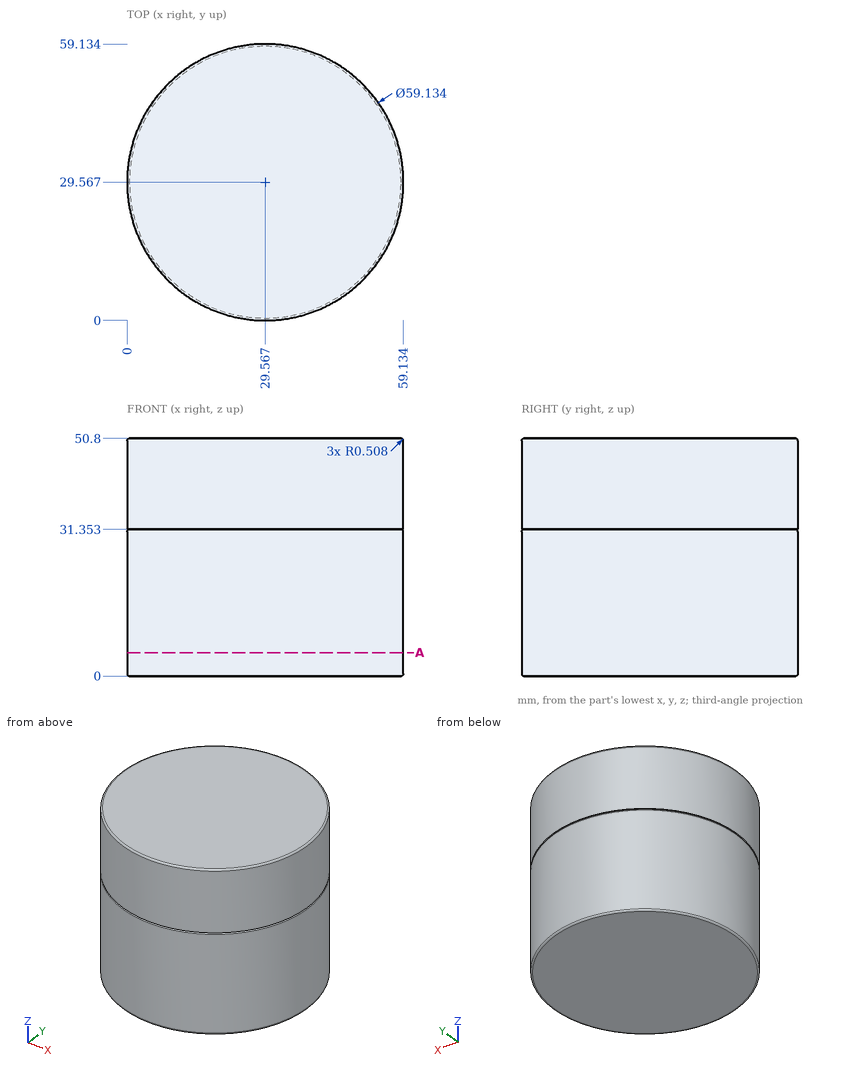
The drawing under review shows one solid part. Ordinate dimensions are in mm from its lowest x, y, z. Give positions to 0.01 mm unless a question says otherwise; leave off trailing zeros. Loops run counter-clockwise (first coordinate to the right, second up) from the corner with the lowest first, then second, coordinate; pieces in that order, holes last. Notation, with made-up numbers: M 87.5,-16 L 92.5,-16 A11 cw 92.5,-11 Z; hole C 44,-23.5 d7. An arc over 180 degrees is marked long. One line per item, written item: value. Start each with the question number.
Q1. For L1, parallel to X at y = 23.5, z = 39.5 (1 decimal); L2, parallel to Y at x = 41, z = 6 (1 decimal); L3, parallel to Y at x = 27, z = 19, list the stretches that pass through material, from the lowest coordinate up.
Q2. Add section A-A (z = 5). Give the boundary of the cut face in (x, y) (1 decimal).
Q3. Clearance check with flat-ended pins moving along their axes: pin 1 Ø12 at (y, z) = (44, 7.5) entering from -X; pin 2 Ø4 at (y, z) = (39.5, 25) entering from +X; pin 3 Ø12 at (x, z) = (48.5, 28) entering from +Y (1 decimal); pin 4 Ø2 at (x, y) = (43.5, 43) entering from -Z. State where each tip first meets the part, or that it passes through.
Reply:
1. L1: 0.6 to 58.5
1. L2: 2.3 to 56.8
1. L3: 0.11 to 59.02
2. outline: C 29.6,29.6 d59.1
3. pin 1: x = 1.23
3. pin 2: x = 58.05
3. pin 3: y = 56.2
3. pin 4: z = 0
